Here's how the part is built. I have some questions about the finished solid (model axes, mm). A direction names the side the tool comes from. Round coordinates to 2 decimals unless told otherwise and drop trailing zeros. Order: outer loops, then holes, each group sorted by start corner. A loop starts at its lowest first (then second) coordinate and runs counter-clockwise, first axis right, second up.
```python
from build123d import *

# Parameters (mm, degrees)
F1_W    = 12.3
F1_H    = 12.3
F1_R    = 4.15
F3_SIZE = 3


with BuildPart() as f2:
    # F2: sweep along a path in F0
    with BuildLine(Plane.XZ) as f2_path:
        Line((0, 0), (20, 0))
        ThreePointArc((20, 0), (27.0710678119, 2.9289321881), (30, 10))
        Line((30, 10), (30, 30))
    # F1 (on Right) → F2 (sweep)
    with BuildSketch(Plane.YZ):
        Rectangle(F1_W, F1_H)
        Circle(F1_R, mode=Mode.SUBTRACT)
    sweep(path=f2_path.line)

    # F3
    f3_edges = [f2.edges().sort_by_distance(p)[0] for p in [
        (23.85, -6.15, 20),
        (36.15, -6.15, 20),
        (36.15, 6.15, 20),
        (23.85, 6.15, 20),
    ]]
    chamfer(f3_edges, length=F3_SIZE)


solid = f2.part
```
1. If we section it at B-B, the plane x = 4: Write out the boundary of the cut face in (y, z), and give its area (3 significant figures).
Evaluation:
outline: (-6.15, -3.15) - (-3.15, -6.15) - (3.15, -6.15) - (6.15, -3.15) - (6.15, 3.15) - (3.15, 6.15) - (-3.15, 6.15) - (-6.15, 3.15) - close; hole circle Ø8.3 at (0, 0)
area: 79.2 mm2
2. If we section it at D-D, the plane y = -5: Write out the boundary of the cut face in (x, z), and give its area (3 significant figures).
Evaluation:
outline: (0, -4.3) - (20, -4.3) arc R14.3 ccw to (34.3, 10) - (34.3, 30) - (25.7, 30) - (25.7, 10) arc R5.7 cw to (20, 4.3) - (0, 4.3) - close
area: 479 mm2
3. On a 3-axis mill with a long thin cutter (end or side, diameter ignored), from which of +Z, -Z, +X, -X, +Y, -Y can I reach the whole of each face in a straight line? I mean faces 1 (the flat face through (25.3, 4.6, 19.9)), 2 (the flat face through (23.85, 0, 20)), 3 (the cylindrical face through (25.885, -0.54, 20.14)), 4 (the flat face through (9.9, -4.6, 4.7)). Say none if no direction works.
Evaluation:
face 1: +Z, -X, +Y
face 2: +Z, -X, +Y, -Y
face 3: +Z
face 4: +Z, -X, -Y
4. If we section it at C-C, the plane z = 16: Write out the boundary of the cut face in (x, y).
Evaluation:
outline: (23.85, -3.15) - (26.85, -6.15) - (33.15, -6.15) - (36.15, -3.15) - (36.15, 3.15) - (33.15, 6.15) - (26.85, 6.15) - (23.85, 3.15) - close; hole circle Ø8.3 at (30, 0)
5. I need wall thicknesses on probe 1 along X at (y, z) = (0, 16.5); probe 2 along Y at (x, z) = (30, 22). Which ranges of each line are inside material? Lowest first, please.
Evaluation:
probe 1: x = 23.85 to 25.85, 34.15 to 36.15
probe 2: y = -6.15 to -4.15, 4.15 to 6.15
6. If we section it at A-A, the plane y = 0: Write out the boundary of the cut face in (x, z), and give its area (3 significant figures).
Evaluation:
outline: (0, -6.15) - (20, -6.15) arc R16.15 ccw to (36.15, 10) - (36.15, 30) - (34.15, 30) - (34.15, 10) arc R14.15 cw to (20, -4.15) - (0, -4.15) - close; (0, 4.15) - (20, 4.15) arc R5.85 ccw to (25.85, 10) - (25.85, 30) - (23.85, 30) - (23.85, 10) arc R3.85 cw to (20, 6.15) - (0, 6.15) - close
area: 223 mm2
7. I'm going to push flat-ended pins straight in: P1, Ø2, axis at y = 4, z = 25, coming from the -X side; P2, Ø3, axis at x = 27, y = 0.5, coming from the -Z side; P3, Ø7, axis at x = 15, y = -0.5, coming from the +Z side. Where does each tip first touch, or does it pass through?
Evaluation:
P1: stops at x = 23.85
P2: stops at z = -5.18
P3: stops at z = 6.15
